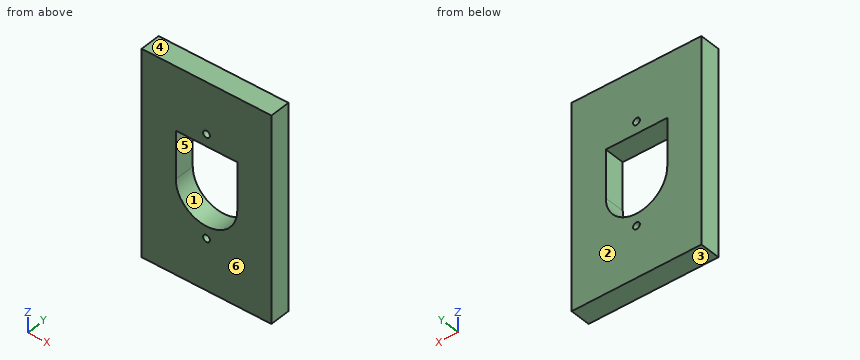
```python
from build123d import *

# Parameters (mm, degrees)
SKETCH1_W           = 19
SKETCH1_H           = 30
BOSS_EXTRUDE1_DEPTH = 3
SKETCH2_R           = 0.5
CUT_EXTRUDE1_DEPTH  = 4


with BuildPart() as part:
    # Sketch1 → Boss-Extrude1 (new body)
    with BuildSketch(Plane(origin=(0, 0, 0), x_dir=(1, 0, 0), z_dir=(0, 1, 0))):
        with Locations((9.5, -15)):
            Rectangle(SKETCH1_W, SKETCH1_H)
    extrude(amount=BOSS_EXTRUDE1_DEPTH)

    # Sketch2 → Cut-Extrude1 (cut, through all)
    with BuildSketch(Plane(origin=(0, 3, 0), x_dir=(1, 0, 0), z_dir=(0, 1, 0))):
        with BuildLine():
            Line((5, -20.75), (14, -20.75))
            Line((14, -20.75), (14, -13.75))
            ThreePointArc((14, -13.75), (9.5, -9.25), (5, -13.75))
            Line((5, -13.75), (5, -20.75))
        make_face()
        with Locations((9.5, -22.5)):
            Circle(SKETCH2_R)
        with Locations((9.5, -7.5)):
            Circle(SKETCH2_R)
    extrude(amount=-CUT_EXTRUDE1_DEPTH, mode=Mode.SUBTRACT)


solid = part.part
```
Can you work these out from the model? Positions are in its coordinate system, mm. Face numbers are marked on the shaded views. A direction names the side the tool comes from. Coordinates: 2 decimals unless noted, no trailing zeros. Write each loop counter-clockwise with the first axis right and the second up, starting at its lowest first coordinate (ties: lowest second). Pieces come first, ordered by that corner, then holes. Notation, with made-up numbers: (-34.5, -31.75) - (-16.5, -31.75) arc R23 ccw to (-16.5, -12.75) - close; hole circle Ø3 at (64.5, 81). An arc over 180 degrees is marked (long way). Return JSON: item names as keys, results as strings.
Q1. If we section it at B-B (y = 1.8): Please give me the cut outline in (x, z), then the cut area to 3 significant figures.
Computed values:
{"outline": "(0, 0) - (19, 0) - (19, 30) - (0, 30) - close; hole (5, 13.75) arc R4.5 ccw to (14, 13.75) - (14, 20.75) - (5, 20.75) - close; hole circle Ø1 at (9.5, 7.5); hole circle Ø1 at (9.5, 22.5)", "area": "474 mm2"}
Q2. On a 3-axis mill with a long thin cutter (end or side, diameter ignored), from which of +Z, -Z, +X, -X, +Y, -Y can I reach the whole of each face in a straight line? I mean the marked faces 5 and 6. Say none if no direction works.
Computed values:
{"face 5": "+Y, -Y", "face 6": "+Z, -Z, +X, -X, -Y"}
Q3. If we section it at C-C (x = 13): Please give me the cut outline in (y, z), then the cut area to 3 significant figures.
Computed values:
{"outline": "(0, 0) - (3, 0) - (3, 10.92) - (0, 10.92) - close; (0, 20.75) - (3, 20.75) - (3, 30) - (0, 30) - close", "area": "60.5 mm2"}
Q4. If we section it at A-A (z = 17.75): Please give me the cut outline in (x, y).
Computed values:
{"outline": "(0, 0) - (5, 0) - (5, 3) - (0, 3) - close; (14, 0) - (19, 0) - (19, 3) - (14, 3) - close"}
Q5. Thinking about a two-plate mould opening in Z: for the marked faces 1, 2, 3 and 4, which applies, +Z half, -Z half, draft (parallel to the pull), parting line (faces both ways), or undercut?
Computed values:
{"face 1": "undercut", "face 2": "draft", "face 3": "-Z half", "face 4": "+Z half"}
Q6. Please list where these lines run through material, in increasing order: L1, parallel to Z at x = 9.5, y = 1.8; L2, parallel to X at y = 2.4, z = 17.5; L3, parallel to X at y = 1.35, z = 7.5. Write a range as from..to.
Computed values:
{"L1": "z = 0..7, 8..9.25, 20.75..22, 23..30", "L2": "x = 0..5, 14..19", "L3": "x = 0..9, 10..19"}
